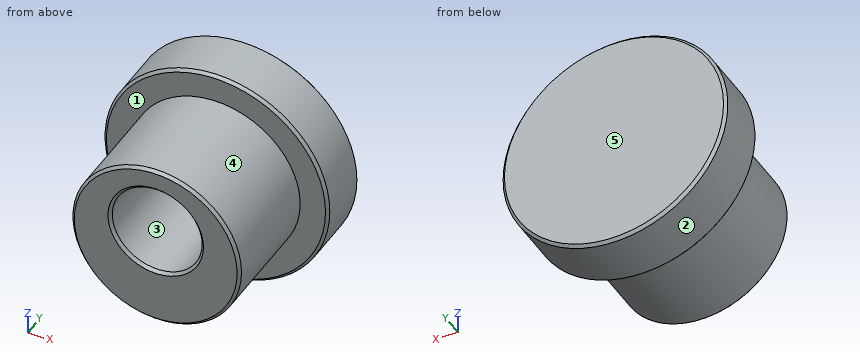
from build123d import *

# Parameters (mm, degrees)
F0_R     = 20
F1_DEPTH = 10
F2_R     = 15
F3_DEPTH = 20
F4_R     = 8
F5_DEPTH = 25
F6_SIZE  = 0.5


with BuildPart() as f1:
    # F0 (on Front) → F1 (new body)
    with BuildSketch(Plane.XZ):
        Circle(F0_R)
    extrude(amount=F1_DEPTH)

    # F2 (on face) → F3 (join)
    with BuildSketch(Plane.XZ.offset(10)):
        Circle(F2_R)
    extrude(amount=F3_DEPTH)

    # F4 (on face) → F5 (cut)
    with BuildSketch(Plane.XZ.offset(30)):
        with Locations((0, 3)):
            Circle(F4_R)
    extrude(amount=-F5_DEPTH, mode=Mode.SUBTRACT)

    # F6
    f6_edges = [f1.edges().sort_by_distance(p)[0] for p in [
        (-15, -30, 0),
        (-20, -10, 0),
        (-20, 0, 0),
        (-8, -30, 3),
    ]]
    chamfer(f6_edges, length=F6_SIZE)


solid = f1.part
Could you check a few things on this model? Use its own coordinates, in mm. Face numbers are marked on the shaded views. A direction names the side the tool comes from. Give positions to 0.01 mm unless a question says otherwise; leave off trailing zeros. Order: outer loops, then holes, each group sorted by start corner. A loop starts at its lowest first (then second) coordinate and runs counter-clockwise, first axis right, second up.
1. Suppose I cut it at B-B (x = 0). List the corners of the cut face in (y, z) for me.
2. I need wall thicknesses on L1, parallel to Z at x = 0, y = -24; L2, parallel to Y at x = 11.5, z = 11; L3, parallel to X at y = -21.5, z = 2. Which ranges of each line are inside material? Lowest first, please.
3. Suppose I cut it at A-A (y = -8.25). List the corners of the cut face in (x, z) for me.
4. For the marked faces 1 and 2, which set-ups out of +Z, -Z, +X, -X, +Y, -Y let a thin tool reach every point of the face, with its end or its side?
5. We'd pull the mould along Z, two halves only. Please class the marked faces 3, 4 and 5: pulls with the +Z half, pulls with the -Z half, needs draft (parallel to the pull), parting line crosses it, or undercut.
6. Will these pins go through, and if not, where does the flat tip stop? P1, Ø8, axis at x = 3.5, z = 1.5, coming from the -Y side; P2, Ø6, axis at y = -16, z = 4.5, coming from the +X side; P3, Ø5, axis at x = -1, y = -14, coming from the -Z side.
7. Suppose I cut it at C-C (y = -26). List the corners of the cut face in (x, z) for me, plus the area to 3 significant figures.
Solved:
1. outline: (-30, -14.5) - (-29.5, -15) - (-10, -15) - (-10, -19.5) - (-9.5, -20) - (-0.5, -20) - (0, -19.5) - (0, 19.5) - (-0.5, 20) - (-9.5, 20) - (-10, 19.5) - (-10, 15) - (-29.5, 15) - (-30, 14.5) - (-30, 11.5) - (-29.5, 11) - (-5, 11) - (-5, -5) - (-29.5, -5) - (-30, -5.5) - close
2. L1: z = -15 to -5, 11 to 15
2. L2: y = -10 to 0
2. L3: x = -14.87 to -7.94, 7.94 to 14.87
3. outline: circle Ø40 at (0, 0); hole circle Ø16 at (0, 3)
4. face 1: -Y
4. face 2: +Y, -Y
5. face 3: undercut
5. face 4: parting line crosses it
5. face 5: needs draft
6. P1: stops at y = -5
6. P2: stops at x = 14.92
6. P3: stops at z = -15
7. outline: circle Ø30 at (0, 0); hole circle Ø16 at (0, 3)
7. area: 506 mm2
